CAD build for the part. Positions are in the model's coordinates, mm. A direction names the side the tool comes from. Give positions to 0.01 mm unless a question says otherwise; leave off trailing zeros. Order: outer loops, then holes, each group sorted by start corner. A loop starts at its lowest first (then second) coordinate and runs counter-clockwise, first axis right, second up.
Item 1: Band-saw the part on A-A on z = -46. Give the cut face in (x, y).
Item 2: Two-plate mould, pull along Y, no slides. Class faces 5 (the flat face through (5, 31, -22)), 6 (the cylindrical face through (15.352, 2.465, -20.526)): released by +Y, released by -Y, zero draft, split by the parting line, or undercut.
Item 3: Which spindle directions (+Z, -Z, +X, -X, +Y, -Y) get a long thin tool onto all of the face, cutting with end or side? Do faces 1 (the flat face through (18, 185, -33)), 2 (the flat face through (7, 182.9, -34)), 3 (the flat face through (5, 64, -22)), 4 (the flat face through (8, 101.9, -2)). Say none if no direction does.
Item 4: Flat gauge pins, fed straight in: P1, Ø1, axis at y = 186, z = -30, coming from the -X side; P2, Ø1, axis at y = 115.5, z = -9.5, coming from the +X side; P3, Ø6.5, axis at x = 7.5, z = -31, coming from the +Y side; P4, Ø6.5, axis at x = 11, z = -3.5, coming from the -Y side. Where does each tip first touch, or does it go through?
Item 5: Wall check: L1, parallel to Y at x = 8.25, z = -28; L2, parallel to Y at x = 6, z = -23; L3, parallel to Y at x = 9.25, z = -26. Give the ranges that are in metal, low to high.
Item 6: Band-saw the part on B-B on z = -55. Give the cut face in (x, y), plus the area to 3 significant figures.
```python
from build123d import *

# Parameters (mm, degrees)
SKETCH1_W           = 25
SKETCH1_H           = 36
BOSS_EXTRUDE1_DEPTH = 186.9
FILLET1_SIZE        = 24
SKETCH2_W           = 5
SKETCH2_H           = 10
CUT_EXTRUDE1_DEPTH  = 4
SKETCH3_W           = 8
SKETCH3_H           = 5.2
SKETCH3_H_2         = 5.6
CUT_EXTRUDE2_DEPTH  = 10
SKETCH4_W           = 41
SKETCH4_H           = 50
BOSS_EXTRUDE2_DEPTH = 2
CUT_EXTRUDE3_REACH  = 202.374
CHAMFER1_SIZE       = 16
SKETCH6_W           = 6
SKETCH6_H           = 4
CUT_EXTRUDE4_DEPTH  = 9
SKETCH7_W           = 3
SKETCH7_H           = 3
CUT_EXTRUDE5_DEPTH  = 10
BOSS_EXTRUDE3_DEPTH = 4
SKETCH9_R           = 2
CUT_EXTRUDE6_DEPTH  = 5
SKETCH10_R          = 1.5
CUT_EXTRUDE7_DEPTH  = 4
SKETCH11_W          = 6
SKETCH11_H          = 16
SKETCH11_H_2        = 20
CUT_EXTRUDE8_DEPTH  = 8
SKETCH12_W          = 10
SKETCH12_H          = 79.7
CUT_EXTRUDE9_DEPTH  = 4
SKETCH13_W          = 10
SKETCH13_H          = 166.9
CUT_EXTRUDE10_DEPTH = 4
SKETCH14_W          = 9
SKETCH14_H          = 6
CUT_EXTRUDE11_DEPTH = 2


with BuildPart() as part:
    # Sketch1 → Boss-Extrude1 (new body)
    with BuildSketch(Plane(origin=(0, 0, 0), x_dir=(1, 0, 0), z_dir=(0, 1, 0))):
        with Locations((12.5, 18)):
            Rectangle(SKETCH1_W, SKETCH1_H)
    extrude(amount=BOSS_EXTRUDE1_DEPTH)

    # Fillet1
    # a fillet whose section is not a circle: 24 mm, written as the material it takes off along each edge
    with BuildSketch(Plane(origin=(25, -60, 0), x_dir=(-1, 0, 0), z_dir=(0, 1, 0))) as fillet1_piece_1:
        with BuildLine():
            Bezier((FILLET1_SIZE, 0), (0, 0), (0, -FILLET1_SIZE), weights=[1, 1.222222222, 1])
            Line((0, -FILLET1_SIZE), (0, 0))
            Line((0, 0), (FILLET1_SIZE, 0))
        make_face()
    extrude(amount=306.9, mode=Mode.SUBTRACT)

    # Sketch2 → Cut-Extrude1 (cut)
    with BuildSketch(Plane.ZY):
        with Locations((-3.7, 78.2)):
            Rectangle(SKETCH2_W, SKETCH2_H)
    extrude(amount=-CUT_EXTRUDE1_DEPTH, mode=Mode.SUBTRACT)

    # Sketch3 → Cut-Extrude2 (cut)
    with BuildSketch(Plane.ZY):
        with Locations((-10, 30.6)):
            Rectangle(SKETCH3_W, SKETCH3_H)
        with Locations((-26, 30.6)):
            Rectangle(SKETCH3_W, SKETCH3_H)
        with Locations((-10, 64)):
            Rectangle(SKETCH3_W, SKETCH3_H_2)
        with Locations((-26, 64)):
            Rectangle(SKETCH3_W, SKETCH3_H_2)
    extrude(amount=-CUT_EXTRUDE2_DEPTH, mode=Mode.SUBTRACT)

    # Sketch4 → Boss-Extrude2 (add)
    with BuildSketch(Plane.ZY):
        with Locations((-46.5, 135)):
            Rectangle(SKETCH4_W, SKETCH4_H)
    extrude(amount=BOSS_EXTRUDE2_DEPTH)

    # Sketch5 → Cut-Extrude3 (cut, up to next)
    with BuildSketch(Plane.ZY.offset(2), mode=Mode.PRIVATE) as cut_extrude3_sk1:
        with BuildLine():
            Line((-59, 131), (-59, 115))
            ThreePointArc((-59, 115), (-61.5, 112.5), (-64, 115))
            Line((-64, 115), (-64, 131))
            ThreePointArc((-64, 131), (-61.5, 133.5), (-59, 131))
        make_face()
    cut_extrude3_tool1 = extrude(cut_extrude3_sk1.sketch, amount=-CUT_EXTRUDE3_REACH, mode=Mode.PRIVATE) & part.part
    # Sketch5 → Cut-Extrude3 (cut, up to next)
    with BuildSketch(Plane.ZY.offset(2), mode=Mode.PRIVATE) as cut_extrude3_sk2:
        with BuildLine():
            Line((-64, 139), (-64, 155))
            ThreePointArc((-64, 155), (-61.5, 157.5), (-59, 155))
            Line((-59, 155), (-59, 139))
            ThreePointArc((-59, 139), (-61.5, 136.5), (-64, 139))
        make_face()
    cut_extrude3_tool2 = extrude(cut_extrude3_sk2.sketch, amount=-CUT_EXTRUDE3_REACH, mode=Mode.PRIVATE) & part.part
    add(cut_extrude3_tool1.solids().sort_by_distance((-2, 123, -61.5))[0], mode=Mode.SUBTRACT)
    add(cut_extrude3_tool2.solids().sort_by_distance((-2, 147, -61.5))[0], mode=Mode.SUBTRACT)

    # Chamfer1
    chamfer1_edges = [part.edges().sort_by_distance(p)[0] for p in [
        (0, 135, -36),
    ]]
    chamfer(chamfer1_edges, length=CHAMFER1_SIZE)

    # Sketch6 → Cut-Extrude4 (cut)
    with BuildSketch(Plane(origin=(0, 0, -36), x_dir=(-1, 0, 0), z_dir=(0, 0, -1))):
        with Locations((-18, 180.9)):
            Rectangle(SKETCH6_W, SKETCH6_H)
        with Locations((-7.2, 180.9)):
            Rectangle(SKETCH6_W, SKETCH6_H)
    extrude(amount=-CUT_EXTRUDE4_DEPTH, mode=Mode.SUBTRACT)

    # Sketch7 → Cut-Extrude5 (cut)
    with BuildSketch(Plane(origin=(0, 186.9, 0), x_dir=(1, 0, 0), z_dir=(0, 1, 0))):
        with Locations((18, 31.5)):
            Rectangle(SKETCH7_W, SKETCH7_H)
        with Locations((7.2, 31.5)):
            Rectangle(SKETCH7_W, SKETCH7_H)
    extrude(amount=-CUT_EXTRUDE5_DEPTH, mode=Mode.SUBTRACT)

    # Sketch8 → Boss-Extrude3 (add)
    with BuildSketch(Plane.XZ):
        Polygon((3, -5), (7, -5), (7, -29), (21, -29), (21, -33), (7, -33), (3, -33), align=None)
    extrude(amount=BOSS_EXTRUDE3_DEPTH)

    # Sketch9 → Cut-Extrude6 (cut)
    with BuildSketch(Plane.XZ):
        with Locations(Location((14, -22, 0), (0, 0, 270))):
            Circle(SKETCH9_R)
    extrude(amount=-CUT_EXTRUDE6_DEPTH, mode=Mode.SUBTRACT)

    # Sketch10 → Cut-Extrude7 (cut)
    with BuildSketch(Plane.XZ):
        with Locations(Location((14, -12, 0), (0, 0, 270))):
            Circle(SKETCH10_R)
    extrude(amount=-CUT_EXTRUDE7_DEPTH, mode=Mode.SUBTRACT)

    # Sketch11 → Cut-Extrude8 (cut)
    with BuildSketch(Plane.XY):
        with Locations((10, 16)):
            Rectangle(SKETCH11_W, SKETCH11_H)
        with Locations((10, 46)):
            Rectangle(SKETCH11_W, SKETCH11_H_2)
    extrude(amount=-CUT_EXTRUDE8_DEPTH, mode=Mode.SUBTRACT)

    # Sketch12 → Cut-Extrude9 (cut)
    with BuildSketch(Plane.XY):
        with Locations((8, 141.75)):
            Rectangle(SKETCH12_W, SKETCH12_H)
    extrude(amount=-CUT_EXTRUDE9_DEPTH, mode=Mode.SUBTRACT)

    # Sketch13 → Cut-Extrude10 (cut)
    with BuildSketch(Plane(origin=(25, 0, 0), x_dir=(0, 0, -1), z_dir=(1, 0, 0))):
        with Locations((31, 93.45)):
            Rectangle(SKETCH13_W, SKETCH13_H)
    extrude(amount=-CUT_EXTRUDE10_DEPTH, mode=Mode.SUBTRACT)

    # Sketch14 → Cut-Extrude11 (cut)
    with BuildSketch(Plane(origin=(0, 186.9, 0), x_dir=(1, 0, 0), z_dir=(0, 1, 0))):
        with Locations((7.2, 30)):
            Rectangle(SKETCH14_W, SKETCH14_H)
        with Locations((18, 30)):
            Rectangle(SKETCH14_W, SKETCH14_H)
    extrude(amount=-CUT_EXTRUDE11_DEPTH, mode=Mode.SUBTRACT)


solid = part.part
```
The answers:
1. outline: (-2, 110) - (6, 110) - (6, 160) - (-2, 160) - close
2. face 5: undercut
2. face 6: zero draft
3. face 1: +Y
3. face 2: -Z
3. face 3: -X
3. face 4: +Z
4. P1: stops at x = 0
4. P2: stops at x = 22.71
4. P3: stops at y = 186.9
4. P4: stops at y = 0
5. L1: y = 0 to 28, 33.2 to 61.2, 66.8 to 178.9, 182.9 to 184.9
5. L2: y = -4 to 28, 33.2 to 61.2, 66.8 to 186.9
5. L3: y = 0 to 28, 33.2 to 61.2, 66.8 to 186.9
6. outline: (-2, 110) - (0, 110) - (0, 160) - (-2, 160) - close
6. area: 100 mm2
